```python
from build123d import *

# Parameters (mm, degrees)
BOSS_EXTRU_1_DEPTH       = 5.6
ENL_V_MAT_EXTRU_1_REACH  = 416.887
ESQUISSE2_W              = 40
ESQUISSE2_H              = 20
ENL_V_MAT_EXTRU_2_REACH  = 416.887
ESQUISSE3_R              = 1.45
SKETCH2_W                = 40
SKETCH2_H                = 20
CUT_EXTRUDE2_DEPTH       = 415.887165384
SKETCH5_R                = 1.45
CUT_EXTRUDE4_DEPTH       = 415.887165384
ESQUISSE4_R              = 1.375
ENL_V_MAT_EXTRU_4_DEPTH  = 415.887165384
ESQUISSE6_R              = 1.45
ENL_V_MAT_EXTRU_6_DEPTH  = 415.887165384
ESQUISSE8_R              = 1.25
ENL_V_MAT_EXTRU_7_DEPTH  = 415.887165384
ESQUISSE9_R              = 1.6
ENL_V_MAT_EXTRU_8_DEPTH  = 415.887165384
ESQUISSE10_W             = 50.45
ESQUISSE10_H             = 75.69
ENL_V_MAT_EXTRU_9_DEPTH  = 415.887165384
ESQUISSE11_W             = 30
ESQUISSE11_H             = 15
ENL_V_MAT_EXTRU_10_DEPTH = 415.887165384
ESQUISSE12_R             = 1.45
ENL_V_MAT_EXTRU_11_DEPTH = 415.887165384
FILLET1_R                = 6.35
FILLET2_R                = 12.7


with BuildPart() as part:
    # Esquisse1 → Boss.-Extru.1 (new body)
    with BuildSketch(Plane.XY):
        Polygon((100, -60), (150, -110), (250, -110), (300, -60), (400, -60), (400, 0), (25.838605695, 0), (0, 0), (0, -60), align=None)
    boss_extru_1 = extrude(amount=BOSS_EXTRU_1_DEPTH)

    # Esquisse2 → Enl_v. mat.-Extru.1 (cut, up to next)
    with BuildSketch(Plane.XY.offset(5.6), mode=Mode.PRIVATE) as enl_v_mat_extru_1_sk1:
        with Locations((50, -50)):
            Rectangle(ESQUISSE2_W, ESQUISSE2_H)
    enl_v_mat_extru_1_tool1 = extrude(enl_v_mat_extru_1_sk1.sketch, amount=-ENL_V_MAT_EXTRU_1_REACH, mode=Mode.PRIVATE) & part.part
    enl_v_mat_extru_1 = enl_v_mat_extru_1_tool1.solids().sort_by_distance((50, -50, 5.6))[0]
    add(enl_v_mat_extru_1, mode=Mode.SUBTRACT)

    # Esquisse3 → Enl_v. mat.-Extru.2 (cut, up to next)
    with BuildSketch(Plane.XY.offset(5.6), mode=Mode.PRIVATE) as enl_v_mat_extru_2_sk1:
        with Locations((26.25, -55.08)):
            Circle(ESQUISSE3_R)
    enl_v_mat_extru_2_tool1 = extrude(enl_v_mat_extru_2_sk1.sketch, amount=-ENL_V_MAT_EXTRU_2_REACH, mode=Mode.PRIVATE) & part.part
    # Esquisse3 → Enl_v. mat.-Extru.2 (cut, up to next)
    with BuildSketch(Plane.XY.offset(5.6), mode=Mode.PRIVATE) as enl_v_mat_extru_2_sk2:
        with Locations((73.75, -55.08)):
            Circle(ESQUISSE3_R)
    enl_v_mat_extru_2_tool2 = extrude(enl_v_mat_extru_2_sk2.sketch, amount=-ENL_V_MAT_EXTRU_2_REACH, mode=Mode.PRIVATE) & part.part
    # Esquisse3 → Enl_v. mat.-Extru.2 (cut, up to next)
    with BuildSketch(Plane.XY.offset(5.6), mode=Mode.PRIVATE) as enl_v_mat_extru_2_sk3:
        with Locations((73.75, -44.92)):
            Circle(ESQUISSE3_R)
    enl_v_mat_extru_2_tool3 = extrude(enl_v_mat_extru_2_sk3.sketch, amount=-ENL_V_MAT_EXTRU_2_REACH, mode=Mode.PRIVATE) & part.part
    # Esquisse3 → Enl_v. mat.-Extru.2 (cut, up to next)
    with BuildSketch(Plane.XY.offset(5.6), mode=Mode.PRIVATE) as enl_v_mat_extru_2_sk4:
        with Locations((26.25, -44.92)):
            Circle(ESQUISSE3_R)
    enl_v_mat_extru_2_tool4 = extrude(enl_v_mat_extru_2_sk4.sketch, amount=-ENL_V_MAT_EXTRU_2_REACH, mode=Mode.PRIVATE) & part.part
    # Esquisse3 → Enl_v. mat.-Extru.2 (cut, up to next)
    with BuildSketch(Plane.XY.offset(5.6), mode=Mode.PRIVATE) as enl_v_mat_extru_2_sk5:
        with Locations((35.06, -29.09)):
            Circle(ESQUISSE3_R)
    enl_v_mat_extru_2_tool5 = extrude(enl_v_mat_extru_2_sk5.sketch, amount=-ENL_V_MAT_EXTRU_2_REACH, mode=Mode.PRIVATE) & part.part
    # Esquisse3 → Enl_v. mat.-Extru.2 (cut, up to next)
    with BuildSketch(Plane.XY.offset(5.6), mode=Mode.PRIVATE) as enl_v_mat_extru_2_sk6:
        with Locations((45.06, -29.09)):
            Circle(ESQUISSE3_R)
    enl_v_mat_extru_2_tool6 = extrude(enl_v_mat_extru_2_sk6.sketch, amount=-ENL_V_MAT_EXTRU_2_REACH, mode=Mode.PRIVATE) & part.part
    enl_v_mat_extru_2_1 = enl_v_mat_extru_2_tool1.solids().sort_by_distance((26.25, -55.08, 5.6))[0]
    add(enl_v_mat_extru_2_1, mode=Mode.SUBTRACT)
    enl_v_mat_extru_2_2 = enl_v_mat_extru_2_tool2.solids().sort_by_distance((73.75, -55.08, 5.6))[0]
    add(enl_v_mat_extru_2_2, mode=Mode.SUBTRACT)
    enl_v_mat_extru_2_3 = enl_v_mat_extru_2_tool3.solids().sort_by_distance((73.75, -44.92, 5.6))[0]
    add(enl_v_mat_extru_2_3, mode=Mode.SUBTRACT)
    enl_v_mat_extru_2_4 = enl_v_mat_extru_2_tool4.solids().sort_by_distance((26.25, -44.92, 5.6))[0]
    add(enl_v_mat_extru_2_4, mode=Mode.SUBTRACT)
    enl_v_mat_extru_2_5 = enl_v_mat_extru_2_tool5.solids().sort_by_distance((35.06, -29.09, 5.6))[0]
    add(enl_v_mat_extru_2_5, mode=Mode.SUBTRACT)
    enl_v_mat_extru_2_6 = enl_v_mat_extru_2_tool6.solids().sort_by_distance((45.06, -29.09, 5.6))[0]
    add(enl_v_mat_extru_2_6, mode=Mode.SUBTRACT)
    enl_v_mat_extru_2 = enl_v_mat_extru_2_1 + enl_v_mat_extru_2_2 + enl_v_mat_extru_2_3 + enl_v_mat_extru_2_4 + enl_v_mat_extru_2_5 + enl_v_mat_extru_2_6  # Enl_v. mat.-Extru.2 as one shape, for the pattern or mirror that repeats it

    # Sketch2 → Cut-Extrude2 (cut, symmetric)
    with BuildSketch(Plane.XY):
        with Locations((350, -50)):
            Rectangle(SKETCH2_W, SKETCH2_H)
        with Locations((200, -100)):
            Rectangle(SKETCH2_W, SKETCH2_H)
    cut_extrude2 = extrude(amount=CUT_EXTRUDE2_DEPTH, both=True, mode=Mode.SUBTRACT)

    # Sketch5 → Cut-Extrude4 (cut, through all)
    with BuildSketch(Plane.XY):
        with Locations((176.25, -105.08)):
            Circle(SKETCH5_R)
        with Locations((223.75, -105.08)):
            Circle(SKETCH5_R)
        with Locations(Location((223.75, -94.92, 0), (0, 0, 180))):
            Circle(SKETCH5_R)
        with Locations(Location((176.25, -94.92, 0), (0, 0, 180))):
            Circle(SKETCH5_R)
        with Locations((326.25, -55.08)):
            Circle(SKETCH5_R)
        with Locations((373.75, -55.08)):
            Circle(SKETCH5_R)
        with Locations(Location((373.75, -44.92, 0), (0, 0, 180))):
            Circle(SKETCH5_R)
        with Locations(Location((326.25, -44.92, 0), (0, 0, 180))):
            Circle(SKETCH5_R)
        with Locations((185.06, -79.09)):
            Circle(SKETCH5_R)
        with Locations((195.06, -79.09)):
            Circle(SKETCH5_R)
        with Locations((335.06, -29.09)):
            Circle(SKETCH5_R)
        with Locations((345.06, -29.09)):
            Circle(SKETCH5_R)
    cut_extrude4 = extrude(amount=CUT_EXTRUDE4_DEPTH, mode=Mode.SUBTRACT)

    # Mirror1: Boss.-Extru.1, Enl_v. mat.-Extru.1, Enl_v. mat.-Extru.2, Cut-Extrude2, Cut-Extrude4 across plane
    add(boss_extru_1.mirror(Plane.ZX))
    add(enl_v_mat_extru_1.mirror(Plane.ZX), mode=Mode.SUBTRACT)
    add(enl_v_mat_extru_2.mirror(Plane.ZX), mode=Mode.SUBTRACT)
    add(cut_extrude2.mirror(Plane.ZX), mode=Mode.SUBTRACT)
    add(cut_extrude4.mirror(Plane.ZX), mode=Mode.SUBTRACT)

    # Esquisse4 → Enl_v. mat.-Extru.4 (cut, through all)
    with BuildSketch(Plane.XY.offset(5.6)):
        with Locations((263, -39)):
            Circle(ESQUISSE4_R)
        with Locations((312, -39)):
            Circle(ESQUISSE4_R)
        with Locations((312, 19)):
            Circle(ESQUISSE4_R)
        with Locations((263, 19)):
            Circle(ESQUISSE4_R)
    extrude(amount=-ENL_V_MAT_EXTRU_4_DEPTH, mode=Mode.SUBTRACT)

    # Esquisse6 → Enl_v. mat.-Extru.6 (cut, through all)
    with BuildSketch(Plane(origin=(0, 0, 0), x_dir=(-1, 0, 0), z_dir=(0, 0, -1))):
        with Locations((-269.19, -26.31)):
            Circle(ESQUISSE6_R)
        with Locations((-305.82, -26.31)):
            Circle(ESQUISSE6_R)
        with Locations((-305.82, 26.52)):
            Circle(ESQUISSE6_R)
        with Locations((-269.19, 26.52)):
            Circle(ESQUISSE6_R)
    extrude(amount=-ENL_V_MAT_EXTRU_6_DEPTH, mode=Mode.SUBTRACT)

    # Esquisse8 → Enl_v. mat.-Extru.7 (cut, through all)
    with BuildSketch(Plane(origin=(0, 0, 0), x_dir=(-1, 0, 0), z_dir=(0, 0, -1))):
        with Locations((-230, 27.95)):
            Circle(ESQUISSE8_R)
        with Locations((-248.8, 27.95)):
            Circle(ESQUISSE8_R)
        with Locations((-248.8, -27.95)):
            Circle(ESQUISSE8_R)
        with Locations((-230, -27.95)):
            Circle(ESQUISSE8_R)
    extrude(amount=-ENL_V_MAT_EXTRU_7_DEPTH, mode=Mode.SUBTRACT)

    # Esquisse9 → Enl_v. mat.-Extru.8 (cut, through all)
    with BuildSketch(Plane(origin=(0, 0, 0), x_dir=(-1, 0, 0), z_dir=(0, 0, -1))):
        with Locations((-153.85903462, -34.88)):
            Circle(ESQUISSE9_R)
        with Locations((-105.63903462, -36.11)):
            Circle(ESQUISSE9_R)
        with Locations((-105.63903462, 46.36)):
            Circle(ESQUISSE9_R)
        with Locations((-153.85903462, 40)):
            Circle(ESQUISSE9_R)
    extrude(amount=-ENL_V_MAT_EXTRU_8_DEPTH, mode=Mode.SUBTRACT)

    # Esquisse10 → Enl_v. mat.-Extru.9 (cut, through all)
    with BuildSketch(Plane(origin=(0, 0, 0), x_dir=(-1, 0, 0), z_dir=(0, 0, -1))):
        with Locations((-192.775, -0.005)):
            Rectangle(ESQUISSE10_W, ESQUISSE10_H)
    extrude(amount=-ENL_V_MAT_EXTRU_9_DEPTH, mode=Mode.SUBTRACT)

    # Esquisse11 → Enl_v. mat.-Extru.10 (cut, through all)
    with BuildSketch(Plane(origin=(0, 0, 0), x_dir=(-1, 0, 0), z_dir=(0, 0, -1))):
        with Locations((-355, 0)):
            Rectangle(ESQUISSE11_W, ESQUISSE11_H)
        with Locations((-65, 0)):
            Rectangle(ESQUISSE11_W, ESQUISSE11_H)
    extrude(amount=-ENL_V_MAT_EXTRU_10_DEPTH, mode=Mode.SUBTRACT)

    # Esquisse12 → Enl_v. mat.-Extru.11 (cut, through all)
    with BuildSketch(Plane.XY.offset(5.6)):
        with Locations((131.819805153, 77.67766953)):
            Circle(ESQUISSE12_R)
        with Locations((114.142135624, 60)):
            Circle(ESQUISSE12_R)
        with Locations(Location((285.857864376, 60, 0), (0, 0, 180))):
            Circle(ESQUISSE12_R)
        with Locations(Location((268.180194847, 77.67766953, 0), (0, 0, 180))):
            Circle(ESQUISSE12_R)
        with Locations((285.857864376, -60)):
            Circle(ESQUISSE12_R)
        with Locations((268.180194847, -77.67766953)):
            Circle(ESQUISSE12_R)
        with Locations(Location((131.819805153, -77.67766953, 0), (0, 0, 180))):
            Circle(ESQUISSE12_R)
        with Locations(Location((114.142135624, -60, 0), (0, 0, 180))):
            Circle(ESQUISSE12_R)
    extrude(amount=-ENL_V_MAT_EXTRU_11_DEPTH, mode=Mode.SUBTRACT)

    # Fillet1
    fillet1_edges = [part.edges().sort_by_distance(p)[0] for p in [
        (0, 60, 2.8),
        (400, 60, 2.8),
        (0, -60, 2.8),
        (400, -60, 2.8),
    ]]
    fillet(fillet1_edges, radius=FILLET1_R)

    # Fillet2
    fillet2_edges = [part.edges().sort_by_distance(p)[0] for p in [
        (100, 60, 2.8),
        (300, 60, 2.8),
        (250, 110, 2.8),
        (150, 110, 2.8),
        (300, -60, 2.8),
        (250, -110, 2.8),
        (150, -110, 2.8),
        (100, -60, 2.8),
    ]]
    fillet(fillet2_edges, radius=FILLET2_R)


solid = part.part
```
The listing builds one solid part. Answer for the finished solid, in the listing's coordinates (mm). Coordinates: 2 decimals unless noted, no trailing zeros. Loops run counter-clockwise (first coordinate to the right, second up) from the corner with the lowest first, then second, coordinate; pieces in that order, holes last. Notation, with made-up numbers: M 63,86.5 L 78,86.5 A20 cw 78,118.5 Z; hole C 33,-6 d11. An arc over 180 degrees is marked long. Answer as a JSON object with one key per item and string values. Group by question number.
Item 1: Section B-B (y = 2) is taken. Write down the section's boundary in (x, z).
Item 2: Section C-C (z = 2.7) is taken. Give the number of separate pieces and of enclosed holes in the cut face, and give its area (3 significant figures).
Item 3: Consider L1, parallel to Y at x = 305.82, z = 3.35; L2, parallel to X at y = 1, z = 1.4; L3, parallel to X at y = 50.5, z = 2.55. Determine where each line is inside the solid, lowest interval first.
Item 4: Section A-A (x = 205.5) is taken. Write down the section's boundary in (y, z), and give its area (3 significant figures).
Item 5: Each of these flat-tipped pins is pushed along its axis until it touches: P1, Ø1.7, axis at x = 19.5, z = 1.5, coming from the +Y side; P2, Ø1.7, axis at x = 373.75, y = -44.92, coming from the -Z side; P3, Ø3, axis at y = 97, z = 3.5, coming from the +X side. Where does it stop, or does it pass through?
Solved:
{
 "1": {"outline": "M 0,0 L 50,0 L 50,5.6 L 0,5.6 Z; M 80,0 L 167.55,0 L 167.55,5.6 L 80,5.6 Z; M 218,0 L 340,0 L 340,5.6 L 218,5.6 Z; M 370,0 L 400,0 L 400,5.6 L 370,5.6 Z"},
 "2": {"separate pieces": "1", "enclosed holes": "63", "area": "53,100 mm2"},
 "3": {"L1": "y = -60 to -27.76, -24.86 to 25.07, 27.97 to 60", "L2": "x = 0 to 50, 80 to 167.55, 218 to 340, 370 to 400", "L3": "x = 0 to 30, 70 to 330, 370 to 400"},
 "4": {"outline": "M -90,0 L -37.85,0 L -37.85,5.6 L -90,5.6 Z; M 37.84,0 L 90,0 L 90,5.6 L 37.84,5.6 Z", "area": "584 mm2"},
 "5": {"P1": "stops at y = 60", "P2": "passes through", "P3": "stops at x = 264.5"}
}
